The figure shows three views and two pictorial views of one solid part (mm, origin at its lowest corner). Answer the questions. A direction names the side the tool comes from. Coordinates: 2 decimals unless noted, no trailing zeros. Write each loop counter-clockwise with the first axis right and the second up, starting at its lowest first coordinate (ties: lowest second). Pieces come first, ordered by that corner, then holes.
Item 1: Section D-D (y = 3.5) is taken. Give the vertices of the cut face in (x, z), then the cut area to 3 significant figures.
Item 2: A tool of negligible diameter and unlimited length cuts with its end or side. For the marked faces 1, 2 and 3, from which of +Z, -Z, +X, -X, +Y, -Y can it reach the whole face along a straight path? Write none if from no direction.
Item 3: Straight lines are drawn through the part: probe 1 along Y at (x, z) = (4, 9.9); probe 2 along X at (y, z) = (24, 6); probe 3 along X at (y, z) = (52.5, 9.2). For each, find the intervals that lie inside material, in ascending order.
Item 4: Determine the mould class of the marked faces 4, 5 and 6 for opening direction Y: released by +Y, released by -Y, zero draft, split by the parting line, or undercut.
Item 5: Each of these flat-tipped pins is pushed along its axis until it touches: P1, Ø0.8, axis at x = 4, y = 52, coming from the +Z side; P2, Ø3.5, axis at y = 5, z = 5.5, coming from the -X side; P3, Ø4, axis at x = 17, z = 3, coming from the -Y side; P4, Ø6, axis at x = 21.5, z = 2.5, coming from the +Y side. Where does it stop, or does it pass through?
Item 6: Section A-A (z = 10.5) is taken. Give the vertices of the cut face in (x, y), then the cut area to 3 significant figures.
Item 7: Section B-B (y = 52.5) is taken. Give the vertices of the cut face in (x, z).
Item 8: Section C-C (x = 17.5) is taken. Give the vertices of the cut face in (y, z), then the cut area to 3 significant figures.
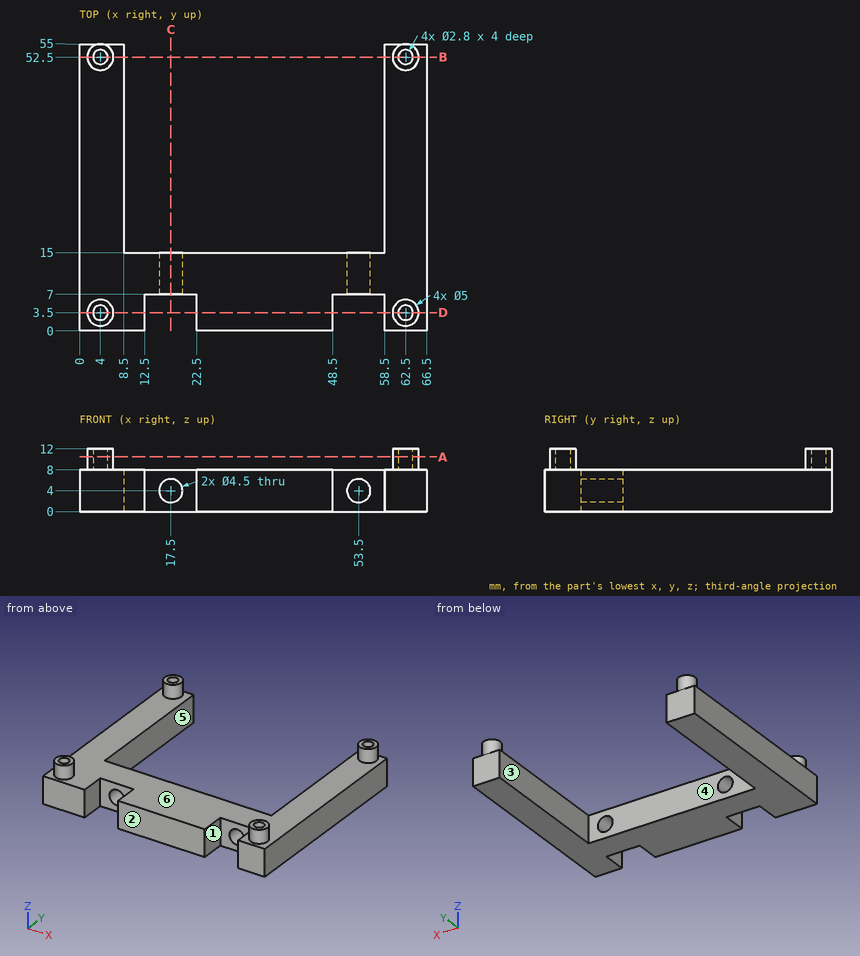
Established:
1. outline: (0, 0) - (12.5, 0) - (12.5, 8) - (6.5, 8) - (6.5, 12) - (5.4, 12) - (5.4, 8) - (2.6, 8) - (2.6, 12) - (1.5, 12) - (1.5, 8) - (0, 8) - close; (22.5, 0) - (48.5, 0) - (48.5, 8) - (22.5, 8) - close; (58.5, 0) - (66.5, 0) - (66.5, 8) - (65, 8) - (65, 12) - (63.9, 12) - (63.9, 8) - (61.1, 8) - (61.1, 12) - (60, 12) - (60, 8) - (58.5, 8) - close
1. area: 390 mm2
2. face 1: +Z, -Z, -Y
2. face 2: +Z, -Z, +X, -X, -Y
2. face 3: +Z, -Z, +Y
3. probe 1: y = 1 to 2.1, 4.9 to 6, 50 to 51.1, 53.9 to 55
3. probe 2: x = 0 to 8.5, 58.5 to 66.5
3. probe 3: x = 1.5 to 2.6, 5.4 to 6.5, 60 to 61.1, 63.9 to 65
4. face 4: released by +Y
4. face 5: zero draft
4. face 6: undercut
5. P1: stops at z = 8
5. P2: stops at x = 0
5. P3: stops at y = 7
5. P4: stops at y = 15
6. outline: circle Ø5 at (4, 3.5); circle Ø5 at (4, 52.5); circle Ø5 at (62.5, 3.5); circle Ø5 at (62.5, 52.5); hole circle Ø2.8 at (4, 3.5); hole circle Ø2.8 at (4, 52.5); hole circle Ø2.8 at (62.5, 3.5); hole circle Ø2.8 at (62.5, 52.5)
6. area: 53.9 mm2
7. outline: (0, 0) - (8.5, 0) - (8.5, 8) - (6.5, 8) - (6.5, 12) - (5.4, 12) - (5.4, 8) - (2.6, 8) - (2.6, 12) - (1.5, 12) - (1.5, 8) - (0, 8) - close; (58.5, 0) - (66.5, 0) - (66.5, 8) - (65, 8) - (65, 12) - (63.9, 12) - (63.9, 8) - (61.1, 8) - (61.1, 12) - (60, 12) - (60, 8) - (58.5, 8) - close
8. outline: (7, 0) - (15, 0) - (15, 1.75) - (7, 1.75) - close; (7, 6.25) - (15, 6.25) - (15, 8) - (7, 8) - close
8. area: 28.0 mm2
